Can you work these out from the model? Positions are in its coordinate system, mm. A direction names the side the tool comes from. Give positions to 0.01 mm unless a question says otherwise; leave off trailing zeros. Order: outer loops, then holes, each group sorted by start corner. A loop starts at its lowest first (then second) coordinate and runs counter-clockwise, first axis right, second up. Notation, with made-up numbers: M 63.5,1.25 L 96.5,1.25 A31 ccw 96.5,37.25 Z; hole C 19.5,17.25 d10. An arc over 180 degrees is marked long. Answer as a JSON object with one key per item and string values.
```python
from build123d import *

# Parameters (mm, degrees)
BASE_FLANGE1_DEPTH = 12.7
CUT_EXTRUDE1_DEPTH = 120.869459796
SCALE1_SCALE       = 0.55


# Sheet-metal steps are written as plain solids
with BuildPart() as part:
    # Sketch2 → Base-Flange1 (new body)
    with BuildSketch(Plane.XY):
        Polygon((0, 0), (7.179503017, 0), (-7.310206248, -25.171495006), (7.689793752, -25.171495006), (22.179503017, 0), (55.200620493, 0), (64.398913039, -25.171495006), (79.398913039, -25.171495006), (70.200620493, 0), (75.200620493, 0), (70.450096018, 13), (65.450096018, 13), (51.553531117, 51.028504994), (36.553531117, 51.028504994), (14.662817791, 13), (9.662817791, 13), (53.353863276, 88.9), (38.353863276, 88.9), (-1.919318718, 18.937505869), (-12.820496983, 0), align=None)
    extrude(amount=-BASE_FLANGE1_DEPTH)

    # Sketch12 → Cut-Extrude1 (cut, through all)
    with BuildSketch(Plane.XY):
        Polygon((29.662817791, 13), (50.450096018, 13), (43.514747433, 31.978858458), (40.587800243, 31.978858458), align=None)
    extrude(amount=-CUT_EXTRUDE1_DEPTH, mode=Mode.SUBTRACT)


with BuildPart() as part_1:
    # Scale1: scaled about (0, 0, 0)
    add(part.part.scale(SCALE1_SCALE))


solid = part_1.part
```
1) I want a section at A-A on y = 24. Write out the boundary of the cut face in (x, z) (3 decimals).
Results found:
{"outline": "M 6.764,-6.985 L 15.014,-6.985 L 15.014,0 L 6.764,0 Z; M 17.764,-6.985 L 29.84,-6.985 L 29.84,0 L 17.764,0 Z"}
2) Thinking about a two-plate mould opening in X: for faces 1 (the face through (8.16, -7.02, -3.44)), 2 (the face through (40.072, 3.525, -3.444)), 3 (the face through (39, -13.844, -3)), which applies, pulls with the +X half, pulls with the -X half, needs draft (parallel to the pull), parting line crosses it, or undercut?
Results found:
{"face 1": "undercut", "face 2": "pulls with the +X half", "face 3": "needs draft"}
3) For faces 4 (the face through (19.36, 12.44, -3.44)), 5 (the face through (41.175, -7.019, -3.444)), 6 (the face through (0.02, -6.825, -3.444)), 7 (the face through (37, 7.15, -3)), which set-ups out of +Z, -Z, +X, -X, +Y, -Y let a thin tool reach every point of the face, with its end or its side?
Results found:
{"face 4": "+Z, -Z", "face 5": "+Z, -Z, +X", "face 6": "+Z, -Z, -X", "face 7": "+Z, -Z, +X, +Y"}
4) I need wall thicknesses on L1, parallel to X at y = 12.5, z = -2.25; L2, parallel to Y at x = 19.5, z = -5.25; L3, parallel to X at y = 17, z = -0.75. Which ranges of each line are inside material? Lowest first, please.
Results found:
{"L1": "x = 0.14 to 8.39, 11.14 to 19.39, 25.79 to 34.04", "L2": "y = 0 to 7.15, 12.68 to 27.02, 31.79 to 46.12", "L3": "x = 2.73 to 10.98, 13.73 to 21.98, 24.15 to 32.4"}
5) I want a section at B-B on x = 39.5. Write out the boundary of the cut face in (y, z) (3 decimals), and give its area (3 significant figures).
Results found:
{"outline": "M -13.844,-6.985 L -2.435,-6.985 L -2.435,0 L -13.844,0 Z; M 0,-6.985 L 5.091,-6.985 L 5.091,0 L 0,0 Z", "area": "115 mm²"}
6) I want a section at D-D on x = 26. Write out the boundary of the cut face in (y, z) (3 decimals), and give its area (3 significant figures).
Results found:
{"outline": "M 0,-6.985 L 7.15,-6.985 L 7.15,0 L 0,0 Z; M 11.932,-6.985 L 28.066,-6.985 L 28.066,0 L 11.932,0 Z; M 43.085,-6.985 L 48.895,-6.985 L 48.895,0 L 43.085,0 Z", "area": "203 mm²"}
7) I want a section at C-C on z = -3. Write out the boundary of the cut face in (x, y) (3 decimals).
Results found:
{"outline": "M -7.051,0 L 3.949,0 L -4.021,-13.844 L 4.229,-13.844 L 12.199,0 L 30.36,0 L 35.419,-13.844 L 43.669,-13.844 L 38.61,0 L 41.36,0 L 38.748,7.15 L 35.998,7.15 L 28.354,28.066 L 20.104,28.066 L 8.065,7.15 L 5.315,7.15 L 29.345,48.895 L 21.095,48.895 Z; hole M 16.315,7.15 L 27.748,7.15 L 23.933,17.588 L 22.323,17.588 Z"}
8) I'm going to push flat-ended pins straight in: pin 1 Ø1 at (x, z) = (17, -1) entering from +Y; pin 2 Ø2 at (x, z) = (21, -2.5) entering from -Y; pin 3 Ø3 at (x, z) = (-0.5, -3.5) entering from +Y. Where does each tip first touch, or does it pass through?
Results found:
{"pin 1": "stops at y = 42.65", "pin 2": "stops at y = 0", "pin 3": "stops at y = 13.99"}
